For this review, take the finished solid that the model builds, in its own axes (mm). Give positions to 0.01 mm unless a question says otherwise; leave off trailing zeros. Loops run counter-clockwise (first coordinate to the right, second up) from the corner with the lowest first, then second, coordinate; pieces in that order, holes last. Notation, with made-up numbers: (0.25, 61) - (16.25, 61) arc R11 ccw to (16.25, 80) - close; hole circle Ø2 at (85.25, -38.5). An arc over 180 degrees is marked (long way). Answer in a Markdown table with one row per item.
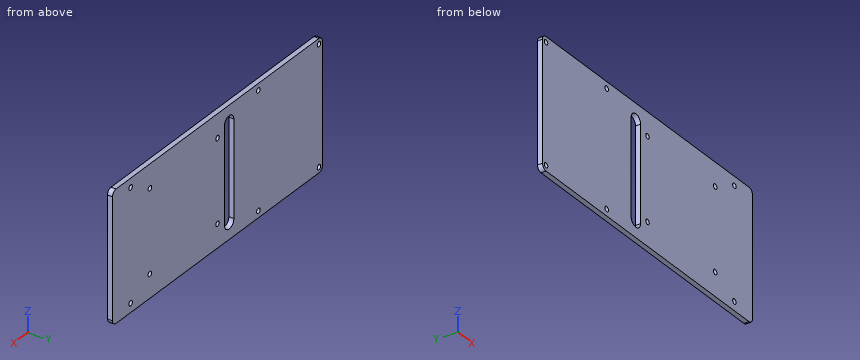
```python
from build123d import *

# Parameters (mm, degrees)
SKETCH1_W           = 180
SKETCH1_H           = 77
SKETCH1_R           = 1.5
SKETCH1_R_2         = 1.500742376
BOSS_EXTRUDE1_DEPTH = 3
FILLET1_R           = 3
SKETCH2_R           = 1.5
CUT_EXTRUDE1_DEPTH  = 3


with BuildPart() as part:
    # Sketch1 → Boss-Extrude1 (new body)
    with BuildSketch(Plane(origin=(0, 0, 0), x_dir=(1, 0, 0), z_dir=(0, 1, 0))):
        Rectangle(SKETCH1_W, SKETCH1_H)
        with Locations(Location((-87, 35.25, 0), (0, 0, 270))):
            Circle(SKETCH1_R, mode=Mode.SUBTRACT)
        with Locations(Location((-87, -35.25, 0), (0, 0, 90))):
            Circle(SKETCH1_R, mode=Mode.SUBTRACT)
        with Locations(Location((-35.005408935, 34.5, 0), (0, 0, 270))):
            Circle(SKETCH1_R, mode=Mode.SUBTRACT)
        with Locations(Location((-35.005408935, -34.5, 0), (0, 0, 90))):
            Circle(SKETCH1_R, mode=Mode.SUBTRACT)
        with Locations(Location((74.494591065, 33.15, 0), (0, 0, 270))):
            Circle(SKETCH1_R_2, mode=Mode.SUBTRACT)
        with Locations(Location((74.494591065, -33.15, 0), (0, 0, 270))):
            Circle(SKETCH1_R, mode=Mode.SUBTRACT)
    extrude(amount=BOSS_EXTRUDE1_DEPTH)

    # Fillet1
    fillet1_edges = [part.edges().sort_by_distance(p)[0] for p in [
        (90, 1.5, 38.5),
        (-90, 1.5, 38.5),
        (-90, 1.5, -38.5),
        (90, 1.5, -38.5),
    ]]
    fillet(fillet1_edges, radius=FILLET1_R)

    # Sketch2 → Cut-Extrude1 (cut)
    with BuildSketch(Plane.XZ):
        with Locations(Location((58, 24.5, 0), (0, 0, 270))):
            Circle(SKETCH2_R)
        with Locations(Location((58, -24.5, 0), (0, 0, 270))):
            Circle(SKETCH2_R)
        with Locations(Location((0, -24.5, 0), (0, 0, 270))):
            Circle(SKETCH2_R)
        with Locations(Location((0, 24.5, 0), (0, 0, 270))):
            Circle(SKETCH2_R)
        with BuildLine():
            Line((-14, 28.5), (-14, -28.5))
            ThreePointArc((-14, -28.5), (-10, -32.5), (-6, -28.5))
            Line((-6, -28.5), (-6, 28.5))
            ThreePointArc((-6, 28.5), (-10, 32.5), (-14, 28.5))
        make_face()
    extrude(amount=-CUT_EXTRUDE1_DEPTH, mode=Mode.SUBTRACT)


solid = part.part
```
1. Wall thickness on line 1 (X direction, y = 2, z = -24.5); line 2 (Z direction, x = -87, y = 1.5); line 3 (X direction, y = 2.3, z = -23.5): over which ranges is each line inside the solid? List them lowest first. Write a range as [from, to].
Values:
| item | result |
|---|---|
| line 1 | x = [-90, -14], [-6, -1.5], [1.5, 56.5], [59.5, 90] |
| line 2 | z = [-38.5, -36.75], [-33.75, 33.75], [36.75, 38.5] |
| line 3 | x = [-90, -14], [-6, -1.12], [1.12, 56.88], [59.12, 90] |
2. We need section A-A, the plane z = 4. Give the boundary of the cut face in (x, y), and give its area (3 significant figures).
Values:
| item | result |
|---|---|
| outline | (-90, 0) - (-14, 0) - (-14, 3) - (-90, 3) - close; (-6, 0) - (90, 0) - (90, 3) - (-6, 3) - close |
| area | 516 mm^2 |
3. Clearance check with a flat-ended pin moving along its axis: pin 1 (4 mm diameter, centred on x = 0, z = -24.5, fed in from +Y). State where the tip first meets the part, or that it passes through.
Values:
| item | result |
|---|---|
| pin 1 | stops at y = 3 |
4. We need section B-B, the plane y = 2. Count the separate pieces of the cut face and the enclosed holes in it, and give its area (3 significant figures).
Values:
| item | result |
|---|---|
| separate pieces | 1 |
| enclosed holes | 11 |
| area | 13,300 mm^2 |
